Can you work these out from the model? Positions are in its coordinate system, mm. Face numbers are marked on the shaded views. A direction names the side the tool comes from. Round coordinates to 2 decimals unless told otherwise and drop trailing zeros. Write each loop counter-clockwise with the first axis right and the second up, starting at its lowest first coordinate (ties: lowest second). Pieces come first, ordered by that corner, then holes.
Q1. Please list where these lines run through material, in increasing order: line 1 along Z through (x, y) = (-314.5, 37); line 2 along X through (y, z) = (9, -140); line 3 along Z through (x, y) = (-254.5, 51).
Q2. If we section it at A-A (z = -145.5): Please give me the cut outline in (x, y).
Q3. For the marked faces 1 and 2, which set-ups out of +Z, -Z, +X, -X, +Y, -Y let a thin tool reach every point of the face, with its end or its side?
Q4. I'm going to push flat-ended pins straight in: pin 1 Ø5.5 at (y, z) = (53, -337.5) entering from -X; pin 2 Ø1.5 at (y, z) = (52.5, -161.5) entering from +X; pin 3 Ø4 at (x, y) = (-292, 54.5) entering from +Z; pin 4 Ø5.5 at (x, y) = (-157.5, 54.5) entering from -Z. Where does each tip first touch, or does it pass through?
Q5. If we section it at C-C (y = 31.5): Please give me the cut outline in (x, z), plus the area to 3 significant figures.
Q6. If we section it at D-D (x = -392): Please give me the cut outline in (y, z).
Q7. If we section it at B-B (x = -281): Please give me the cut outline in (y, z), plus the area to 3 significant figures.
Autodesk Inventor part; units mm, degrees
ref_plane "YZ Plane" through (0, 0, 0) normal (1, 0, 0) x (0, 1, 0)
ref_plane "XZ Plane" through (0, 0, 0) normal (0, 1, 0) x (-1, 0, 0)
ref_plane "XY Plane" through (0, 0, 0) normal (0, 0, 1) x (1, 0, 0)
sketch "Sketch1" plane through (0, 0, 0) normal (0, 1, 0) x (-1, 0, 0)
  line L0 (0, 0) -> (460, 0)
  line L1 (460, 0) -> (460, -507)
  line L2 (460, -507) -> (0, -507)
  line L3 (0, -507) -> (0, 0)
  line L4 (331.3, -133.5) -> (141.3, -133.5)
  line L5 (141.3, -133.5) -> (141.3, -373.5)
  line L6 (141.3, -373.5) -> (331.3, -373.5)
  line L7 (331.3, -373.5) -> (331.3, -133.5)
  dimension "d0" = 460
  dimension "d1" = 507
  dimension "d2" = 190
  dimension "d3" = 240
  dimension "d4" = 133.5
  dimension "d5" = 141.3
extrude "Extrusion1" add sketch "Sketch1" along normal blind 50.8
sketch "Sketch5" plane through (0, 50.8, 0) normal (0, 1, 0) x (1, 0, 0)
  line L0 (-408, 54) -> (-56, 54)
  line L1 (-56, 54) -> (-56, 453)
  line L2 (-56, 453) -> (-408, 453)
  line L3 (-408, 453) -> (-408, 54)
  line L4 (-460, 0) -> (0, 0)
  line L5 (-460, 507) -> (-460, 0)
  line L6 (-331.3, 133.5) -> (-141.3, 133.5)
  line L7 (-141.3, 373.5) -> (-331.3, 373.5)
  line L8 (-331.3, 133.5) -> (-141.3, 133.5)
  line L9 (-141.3, 133.5) -> (-141.3, 373.5)
  line L10 (-141.3, 373.5) -> (-331.3, 373.5)
  line L11 (-331.3, 373.5) -> (-331.3, 133.5)
  dimension "d14" = 352
  dimension "d15" = 399
  dimension "d16" = 54
  dimension "d17" = 52
extrude "Extrusion2" add sketch "Sketch5" along normal blind 5
properties part number "TapaFrontal"
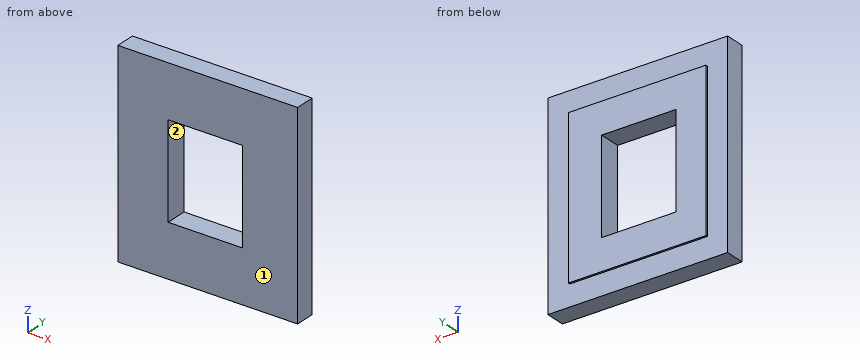
A:
1. line 1: z = -507 to -373.5, -133.5 to 0
1. line 2: x = -460 to -331.3, -141.3 to 0
1. line 3: z = -453 to -373.5, -133.5 to -54
2. outline: (-460, 0) - (-331.3, 0) - (-331.3, 55.8) - (-408, 55.8) - (-408, 50.8) - (-460, 50.8) - close; (-141.3, 0) - (0, 0) - (0, 50.8) - (-56, 50.8) - (-56, 55.8) - (-141.3, 55.8) - close
3. face 1: +Z, -Z, +X, -X, -Y
3. face 2: +Y, -Y
4. pin 1: stops at x = -460
4. pin 2: stops at x = -56
4. pin 3: stops at z = -54
4. pin 4: stops at z = -453
5. outline: (-460, -507) - (0, -507) - (0, 0) - (-460, 0) - close; hole (-331.3, -373.5) - (-141.3, -373.5) - (-141.3, -133.5) - (-331.3, -133.5) - close
5. area: 188,000 mm2
6. outline: (0, -507) - (50.8, -507) - (50.8, -453) - (55.8, -453) - (55.8, -54) - (50.8, -54) - (50.8, 0) - (0, 0) - close
7. outline: (0, -507) - (50.8, -507) - (50.8, -453) - (55.8, -453) - (55.8, -373.5) - (0, -373.5) - close; (0, -133.5) - (55.8, -133.5) - (55.8, -54) - (50.8, -54) - (50.8, 0) - (0, 0) - close
7. area: 14,400 mm2
